from build123d import *

# Parameters (mm, degrees)
SKETCH1_R           = 174.85
SKETCH1_R_2         = 3.556
SKETCH1_R_3         = 162.15
BOSS_EXTRUDE1_DEPTH = 3.175
CUT_EXTRUDE1_DEPTH  = 4.175


with BuildPart() as part:
    # Sketch1 → Boss-Extrude1 (new body)
    with BuildSketch(Plane(origin=(0, 0, 0), x_dir=(1, 0, 0), z_dir=(0, 1, 0))):
        Circle(SKETCH1_R)
        with Locations((0, 168.5)):
            Circle(SKETCH1_R_2, mode=Mode.SUBTRACT)
        with Locations((145.925280538, 84.25)):
            Circle(SKETCH1_R_2, mode=Mode.SUBTRACT)
        with Locations((145.925280538, -84.25)):
            Circle(SKETCH1_R_2, mode=Mode.SUBTRACT)
        with Locations((0, -168.5)):
            Circle(SKETCH1_R_2, mode=Mode.SUBTRACT)
        with Locations((-145.925280538, -84.25)):
            Circle(SKETCH1_R_2, mode=Mode.SUBTRACT)
        with Locations((-145.925280538, 84.25)):
            Circle(SKETCH1_R_2, mode=Mode.SUBTRACT)
        Circle(SKETCH1_R_3, mode=Mode.SUBTRACT)
    extrude(amount=BOSS_EXTRUDE1_DEPTH)

    # Sketch2 → Cut-Extrude1 (cut, through all)
    with BuildSketch(Plane(origin=(0, 0, 0), x_dir=(1, 0, 0), z_dir=(0, 1, 0))):
        with BuildLine():
            Line((-88.9, 153.979316793), (-84.25, 145.925280538))
            ThreePointArc((-84.25, 145.925280538), (-77.80464133, 149.461325391), (-71.211177103, 152.712862116))
            Line((-71.211177103, 152.712862116), (-68.527551141, 146.957807668))
            ThreePointArc((-68.527551141, 146.957807668), (-74.872537636, 143.8288066), (-81.075, 140.426019224))
            Line((-81.075, 140.426019224), (0, 0))
            Line((0, 0), (-81.075, -140.426019224))
            ThreePointArc((-81.075, -140.426019224), (-87.123131493, -136.755922939), (-93.005419154, -132.825503981))
            Line((-93.005419154, -132.825503981), (-96.647629525, -138.027119463))
            ThreePointArc((-96.647629525, -138.027119463), (-90.534984006, -142.111458619), (-84.25, -145.925280538))
            Line((-84.25, -145.925280538), (-87.425, -151.424541852))
            Line((-87.425, -151.424541852), (-88.9, -153.979316793))
            ThreePointArc((-88.9, -153.979316793), (177.8, 0), (-88.9, 153.979316793))
        make_face()
    extrude(amount=CUT_EXTRUDE1_DEPTH, mode=Mode.SUBTRACT)


solid = part.part
Geometry: final body of the model. Coordinates: model frame, mm. A direction names the side the tool comes from. Coordinates: 2 decimals unless noted, no trailing zeros. Order: outer loops, then holes, each group sorted by start corner. A loop starts at its lowest first (then second) coordinate and runs counter-clockwise, first axis right, second up. Notation, with made-up numbers: (83, 85) - (130, 85) arc R11 ccw to (130, 90) - close; hole circle Ø10 at (4, 57.25). An arc over 180 degrees is marked (long way). Use one line per item in the form item = value.
1) Section A-A (y = 2.55). State how many separate pieces and enclosed holes the cut face has, then the cut area to 3 significant figures.
Solutions:
separate_pieces = 1
enclosed_holes = 2
area = 4,400 mm^2
2) Mould query, pull axis Z, two halves, no side actions, for faces 4 (the face through (-174.83, 1.57, -2.56)), 5 (the face through (-165, 0, -1)), 6 (the face through (-149.478, 1.565, -84.406)). Classes: +Z half, -Z half, draft (parallel to the pull), parting line (faces both ways), or undercut.
Solutions:
face_4 = parting line
face_5 = draft
face_6 = undercut
3) Section B-B (x = -129.5). Return loops of the section in (y, z) (3 decimals), then the cut area to 3 significant figures.
Solutions:
outline = (0, -117.483) - (3.175, -117.483) - (3.175, -97.583) - (0, -97.583) - close; (0, 97.583) - (3.175, 97.583) - (3.175, 117.483) - (0, 117.483) - close
area = 126 mm^2
4) Section D-D (z = -26). Return loops of the section in (x, y) (3 decimals).
Solutions:
outline = (-172.906, 0) - (-160.052, 0) - (-160.052, 3.175) - (-172.906, 3.175) - close
5) Section C-C (z = -84.25). Return loops of the section in (x, y) (3 decimals).
Solutions:
outline = (-153.214, 0) - (-149.481, 0) - (-149.481, 3.175) - (-153.214, 3.175) - close; (-142.369, 0) - (-138.544, 0) - (-138.544, 3.175) - (-142.369, 3.175) - close
6) Set-up query: faces 1 (the face through (-77.9, 1.57, -149.41)), 2 (the face through (-165, 3.175, -1)), 3 (the face through (-90.622, 1.565, 142.056)). Return all of +Z, -Z, +X, -X, +Y, -Y with unobstructed straight access to the full face (end or side cutting, diameter ignored); none if empty.
Solutions:
face_1 = -Z, +Y, -Y
face_2 = +Z, -Z, +X, -X, +Y
face_3 = +X, +Y, -Y
7) Ray query, L1, parallel to Z at x = -94, y = 2.5; L2, parallel to Z at x = -146, y = 3; L3, parallel to X at y = 0.9, z = 84.25. Return the intervals inside material, ascending.
Solutions:
L1 = -147.43 to -132.12, 132.12 to 134.25, 139.84 to 147.43
L2 = -96.21 to -87.81, -80.69 to -70.55, 70.55 to 80.69, 87.81 to 96.21
L3 = -153.21 to -149.48, -142.37 to -138.54
8) Pin query (flat end, axial travel): pin 1 (10 mm diameter, centred on x = -153.5, z = -36, fed in from +Y) (3 decimals); pin 2 (2 mm diameter, centred on x = -114.5, z = 112, fed in from -Y); pin 3 (1 mm diameter, centred on y = 0.5, z = -110, fed in from +X). Return the tip coordinate at first contact, or that it passes through.
Solutions:
pin_1 = 3.175
pin_2 = through
pin_3 = -118.67
